Autodesk Inventor part; units mm, degrees
ref_plane "Work Plane1" through (1.525, 0, 0) normal (0, 0, 1) x (1, 0, 0)
ref_plane "YZ Plane" through (0, 0, 0) normal (1, 0, 0) x (0, 1, 0)
ref_plane "XZ Plane" through (0, 0, 0) normal (0, 1, 0) x (-1, 0, 0)
sketch "Sketch1" plane through (0, 0, 0) normal (0, 0, 1) x (1, 0, 0)
  line L0 (0, 16.805) -> (0, 12)
  line L1 (9, 12) -> (45, 12)
  line L2 (45, 12) -> (45, 0)
  line L3 (45, 0) -> (-0.8001, 0)
  line L4 (-9.9601, 0) -> (54.16, 0)
  line L5 (-0.8001, 0) -> (-0.8001, 16.805)
  line L6 (-0.8001, 16.805) -> (0, 16.805)
  line L7 (9, 12) -> (7.1596, 12)
  line L8 (7.1596, 12) -> (0, 12)
  line L9 (0, -3.361) -> (0, 20.166)
  dimension "d0" = 45
  dimension "d1" = 36
  dimension "d2" = 24
  dimension "d9" = 0.8001
  dimension "d10" = 33.61
  dimension "d13" = 1.8404
  dimension "d14" = 24
revolve "Body" add sketch "Sketch1" angle 360 about axis through (45, 0, 0) along (-1, 0, 0)
sketch "Sketch2" plane through (-0.8001, 0, 0) normal (-1, 0, 0) x (0, 0, 1)
  line L0 (0, 20.7846) -> (18, 10.3923)
  line L1 (18, 10.3923) -> (18, -10.3923)
  line L2 (18, -10.3923) -> (0, -20.7846)
  line L3 (0, -20.7846) -> (-18, -10.3923)
  line L4 (-18, -10.3923) -> (-18, 10.3923)
  line L5 (-18, 10.3923) -> (0, 20.7846)
  point P0 (0, 0)
  point P1 (0, 0)
  dimension "d11" = 36
extrude "Head" add sketch "Sketch2" along normal blind 14.2
sketch "Sketch4" plane through (0, 0, 0) normal (0, 0, 1) x (1, 0, 0)
  line L0 (-15.0001, 18) -> (-15.0001, 20.7846)
  line L1 (-15.0001, 20.7846) -> (-13.3924, 20.7846)
  line L2 (-13.3924, 20.7846) -> (-15.0001, 18)
  line L3 (-17.8401, 0) -> (2.0399, 0)
  line L4 (-0.8001, 20.7846) -> (-15.0001, 20.7846)
  line L5 (-15.0001, 10.3923) -> (-15.0001, 20.7846)
  dimension "d5" = 30
  dimension "d19" = 36
revolve "Chamfer1" cut sketch "Sketch4" angle 360 about axis through (-10, 0, 0) along (1, 0, 0)
thread "Thread"
chamfer "Chamfer2" distance 1.8403 distance2 1.8405 1 edges at (45, -12, 0) measured on face at (45, -4.6056, 1.5967)
ref_plane "Work Plane1" through (1.525, 0, 0) normal (0, 0, 1) x (1, 0, 0)
equation "\"d0\" = NLG"
equation "\"d1\" = GEL"
equation "\"d2\" = GD"
equation "\"d10\" = SD2"
equation "\"d14\" = BDM"
equation "\"d11\" = SW"
equation "\"d3\" = KOH - SD"
equation "\"d5\" = ANG1"
equation "\"d19\" = SW0"
equation "\"d15\" = GEL"
equation "\"d6\" = -0.5 * SPD + 0.5 * GD"
equation "\"NLG\" = 45"
equation "\"GD\" = NND"
equation "\"BDM\" = NND"
equation "\"KOH\" = 15"
equation "\"GEL\" = 36"
equation "\"SW\" = 36"
equation "\"SW0\" = SW"
equation "\"SPD\" = NND - 1.2269 * PTC"
equation "\"SD2\" = SDH"
equation "\"SD\" = 0.8"
equation "\"ANG1\" = 30deg"
equation "\"GAL\" = 0.61345 * PTC"
equation "\"GUL\" = 0.61345 * PTC"
equation "\"RR\" = 0.8"
equation "\"GD1\" = THREADDIA - 1.2269 * PTC"
equation "\"THREADDIA\" = 24"
equation "\"SDH\" = 33.61"
equation "\"SDHG\" = 9"
equation "\"TOA\" = 30deg"
equation "\"PTC\" = 3"
equation "\"NND\" = 24"
equation "\"E0\" = 1.155 * SW"
properties part number "JIS B 1180 - A + B M24x45" material "Steel, Mild"
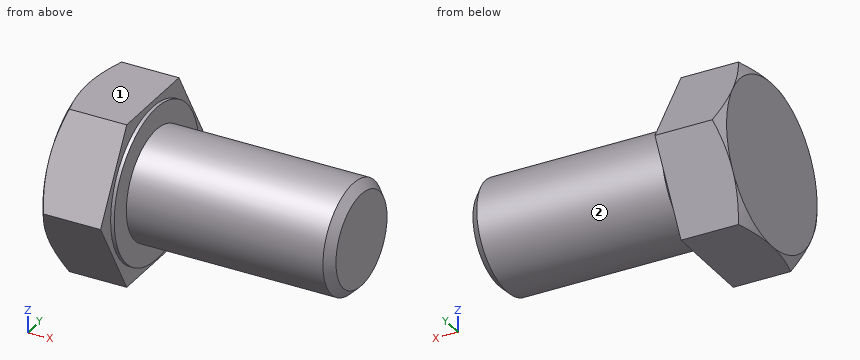
Verification items for the finished model (mm, model axes). Face numbers are marked on the shaded views. A direction names the side the tool comes from. Round coordinates to 2 decimals unless told otherwise and drop trailing zeros. Order: outer loops, then holes, each group sorted by start corner. A loop starts at its lowest first (then second) coordinate and runs counter-clockwise, first axis right, second up.
1. Go/stop test with flat-tipped pins: P1, Ø1, axis at x = 6, z = -5.5, coming from the +Y side; P2, Ø4, axis at y = 11.5, z = -9.5, coming from the +X side; P3, Ø5, axis at x = 14.5, y = -13.5, coming from the +Z side. Record where each tip stops, or that it passes through.
Final values:
P1: stops at y = 10.91
P2: stops at x = 0
P3: stops at z = 4.8
2. Section check B-B on x = 16. Record the cut outline in (y, z).
Final values:
outline: circle Ø24 at (0, 0)
3. Thickness scan on L1, parallel to X at y = 12.5, z = -7; L2, parallel to X at y = 14.5, z = 10; L3, parallel to Y at x = 42.5, z = -10.5. Record the ranges inside material, lowest first.
Final values:
L1: x = -15 to 0
L2: x = -15 to -0.8
L3: y = -5.81 to 5.81
4. Access from +Z, -Z, +X, -X, +Y, -Y to the whole of each face (thin tool, end or side, straight path). Record for the marked faces 1 and 2.
Final values:
face 1: +Z, +X, -X, +Y, -Y
face 2: +X
5. Section check A-A on x = -10.5. Record the cut outline in (y, z).
Final values:
outline: (-20.78, 0) - (-10.39, -18) - (10.39, -18) - (20.78, 0) - (10.39, 18) - (-10.39, 18) - close
